```python
from build123d import *

# Parameters (mm, degrees)
F1_W     = 30
F1_H     = 30
F1_W_2   = 10
F1_H_2   = 10
F2_DEPTH = 30
F3_W     = 10
F3_H     = 10
F4_DEPTH = 30
F5_W     = 10
F5_H     = 10
F6_DEPTH = 30


with BuildPart() as f2:
    # F1 (on Top) → F2 (new body)
    with BuildSketch(Plane.XY):
        Rectangle(F1_W, F1_H)
        Rectangle(F1_W_2, F1_H_2, mode=Mode.SUBTRACT)
    extrude(amount=F2_DEPTH)

    # F3 (on face) → F4 (cut, through all)
    with BuildSketch(Plane(origin=(0, 15, 0), x_dir=(-1, 0, 0), z_dir=(0, 1, 0))):
        with Locations((0, 15)):
            Rectangle(F3_W, F3_H)
    extrude(amount=-F4_DEPTH, mode=Mode.SUBTRACT)

    # F5 (on face) → F6 (cut, through all)
    with BuildSketch(Plane(origin=(-15, 0, 0), x_dir=(0, -1, 0), z_dir=(-1, 0, 0))):
        with Locations((0, 15)):
            Rectangle(F5_W, F5_H)
    extrude(amount=-F6_DEPTH, mode=Mode.SUBTRACT)


solid = f2.part
```
The listing builds one solid part. Answer for the finished solid, in the listing's coordinates (mm). A direction names the side the tool comes from. Give positions to 0.01 mm unless a question says otherwise; leave off trailing zeros. Write each loop counter-clockwise with the first axis right and the second up, starting at its lowest first coordinate (ties: lowest second). Pieces come first, ordered by that corner, then holes. Notation, with made-up numbers: (-31, 34) - (-6, 34) arc R28 cw to (-6, 55) - close; hole circle Ø8 at (-11.5, 9). An arc over 180 degrees is marked (long way). Use one line per item in the form item = value. Start each with the question number.
1) A tool of negligible diameter and unlimited length cuts with its end or side. For faces 1 (the face through (15, 0, 8)), 2 (the face through (0, -15, 8)), 3 (the face through (0, -5, 5)), 4 (the face through (10, -5, 15)), 5 (the face through (-5, 10, 15)), from which of +Z, -Z, +X, -X, +Y, -Y can it reach the whole face along a straight path? Write none if from no direction.
2) Find section A-A on z = 15.75. Determine the outline of the cut face in (x, y), plus the area to 3 significant figures.
3) The mould has two halves that part along X. Classify faces 6 (the face through (5, 0, 5)), 7 (the face through (-15, 0, 8)), 8 (the face through (-7, 0, 0)): pulls with the +X half, pulls with the -X half, needs draft (parallel to the pull), parting line crosses it, or undercut.
4) Consider line 1 along X through (y, z) = (-10.75, 15.5); line 2 along Z through (x, y) = (-11.5, -1.75). Determine where each line is inside the solid, lowest interval first. Write a range as from..to.
5) Find section C-C on y = 13. Determine the outline of the cut face in (x, z).
6) Find section D-D on z = 21.25. Determine the outline of the cut face in (x, y).
7) Find section B-B on x = -1.25. Determine the outline of the cut face in (y, z).
Geometry results:
q1.face_1 = +Z, -Z, +X, +Y, -Y
q1.face_2 = +Z, -Z, +X, -X, -Y
q1.face_3 = +Z, -Z
q1.face_4 = +X, -X
q1.face_5 = +Y, -Y
q2.outline = (-15, -15) - (-5, -15) - (-5, -5) - (-15, -5) - close; (-15, 5) - (-5, 5) - (-5, 15) - (-15, 15) - close; (5, -15) - (15, -15) - (15, -5) - (5, -5) - close; (5, 5) - (15, 5) - (15, 15) - (5, 15) - close
q2.area = 400 mm2
q3.face_6 = undercut
q3.face_7 = pulls with the -X half
q3.face_8 = needs draft
q4.line_1 = -15..-5, 5..15
q4.line_2 = 0..10, 20..30
q5.outline = (-15, 0) - (15, 0) - (15, 30) - (-15, 30) - close; hole (-5, 10) - (5, 10) - (5, 20) - (-5, 20) - close
q6.outline = (-15, -15) - (15, -15) - (15, 15) - (-15, 15) - close; hole (-5, -5) - (5, -5) - (5, 5) - (-5, 5) - close
q7.outline = (-15, 0) - (-5, 0) - (-5, 10) - (-15, 10) - close; (-15, 20) - (-5, 20) - (-5, 30) - (-15, 30) - close; (5, 0) - (15, 0) - (15, 10) - (5, 10) - close; (5, 20) - (15, 20) - (15, 30) - (5, 30) - close
